Can you work these out from the model? Positions are in its coordinate system, mm. Face numbers are marked on the shaded views. A direction names the side the tool comes from. Give positions to 0.01 mm unless a question says otherwise; leave off trailing zeros. Order: outer loops, then holes, each group sorted by start corner. A loop starts at its lowest first (then second) coordinate and runs counter-clockwise, first axis right, second up. Notation, with made-up numbers: (-11, 75) - (36, 75) arc R22 ccw to (36, 99) - close; hole circle Ø7 at (2, 46.5). An arc over 180 degrees is marked (long way). Answer as CSV lines item,"result".
```python
from build123d import *

# Parameters (mm, degrees)
SKETCH1_R           = 1
BOSS_EXTRUDE1_DEPTH = 3
SKETCH2_W           = 15
SKETCH2_H           = 25
CUT_EXTRUDE1_DEPTH  = 1
SKETCH3_W           = 15
SKETCH3_H           = 25
CUT_EXTRUDE2_DEPTH  = 1


with BuildPart() as part:
    # Sketch1 → Boss-Extrude1 (new body)
    with BuildSketch(Plane(origin=(0, 0, 0), x_dir=(1, 0, 0), z_dir=(0, 1, 0))):
        with BuildLine():
            Line((-52.254901961, 26.274509804), (-12.254901961, 26.274509804))
            ThreePointArc((-12.254901961, 26.274509804), (-8.719368055, 24.81004371), (-7.254901961, 21.274509804))
            Line((-7.254901961, 21.274509804), (-7.254901961, -28.725490196))
            ThreePointArc((-7.254901961, -28.725490196), (-8.719368055, -32.261024102), (-12.254901961, -33.725490196))
            Line((-12.254901961, -33.725490196), (-52.254901961, -33.725490196))
            ThreePointArc((-52.254901961, -33.725490196), (-55.790435867, -32.261024102), (-57.254901961, -28.725490196))
            Line((-57.254901961, -28.725490196), (-57.254901961, 21.274509804))
            ThreePointArc((-57.254901961, 21.274509804), (-55.790435867, 24.81004371), (-52.254901961, 26.274509804))
        make_face()
        with Locations(Location((-32.254901961, -3.725490196, 0), (0, 0, 270))):
            Circle(SKETCH1_R, mode=Mode.SUBTRACT)
        with Locations(Location((-47.254901961, 3.774509804, 0), (0, 0, 270))):
            Circle(SKETCH1_R, mode=Mode.SUBTRACT)
        with Locations(Location((-47.254901961, -11.225490196, 0), (0, 0, 270))):
            Circle(SKETCH1_R, mode=Mode.SUBTRACT)
        with Locations(Location((-17.254901961, 3.774509804, 0), (0, 0, 270))):
            Circle(SKETCH1_R, mode=Mode.SUBTRACT)
        with Locations(Location((-17.254901961, -11.225490196, 0), (0, 0, 270))):
            Circle(SKETCH1_R, mode=Mode.SUBTRACT)
    extrude(amount=BOSS_EXTRUDE1_DEPTH)

    # Sketch2 → Cut-Extrude1 (cut)
    with BuildSketch(Plane(origin=(0, 3, 0), x_dir=(1, 0, 0), z_dir=(0, 1, 0))):
        with Locations((-49.754901961, -3.725490196)):
            Rectangle(SKETCH2_W, SKETCH2_H)
    extrude(amount=-CUT_EXTRUDE1_DEPTH, mode=Mode.SUBTRACT)

    # Sketch3 → Cut-Extrude2 (cut)
    with BuildSketch(Plane(origin=(0, 3, 0), x_dir=(1, 0, 0), z_dir=(0, 1, 0))):
        with Locations((-14.754901961, -3.725490196)):
            Rectangle(SKETCH3_W, SKETCH3_H)
    extrude(amount=-CUT_EXTRUDE2_DEPTH, mode=Mode.SUBTRACT)


solid = part.part
```
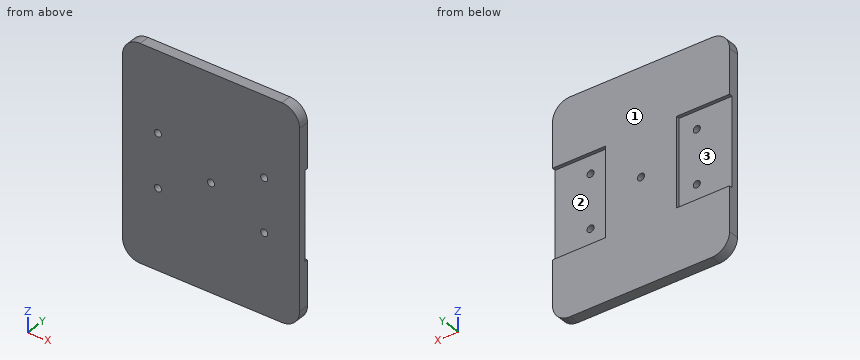
1) Which directions (+Z, -Z, +X, -X, +Y, -Y) give clear straight access to the entire face, cutting with the end or side of a thin tool? Please do the marked faces 1, 2 and 3.
Answer block:
face 1,"+Z, -Z, +X, -X, +Y"
face 2,"+X, +Y"
face 3,"-X, +Y"
2) I need wall thicknesses on line 1 along Z through (x, y) = (-17, 2.6); line 2 along X through (y, z) = (2.1, -8.5); line 3 along Z through (x, y) = (-46.5, 0.7). Which ranges of each line are inside material? Lowest first, please. Write a range as [from, to].
Answer block:
line 1,"[-26.27, -8.77], [16.23, 33.73]"
line 2,"[-42.25, -22.25]"
line 3,"[-26.27, -4.43], [-3.12, 10.57], [11.88, 33.73]"
3) I want a section at B-B on x = -49.5. Write out the boundary of the cut face in (y, z), plus the area to 3 significant figures.
Answer block:
outline,"(0, -26.27) - (3, -26.27) - (3, -8.77) - (2, -8.77) - (2, 16.23) - (3, 16.23) - (3, 33.73) - (0, 33.73) - close"
area,"155 mm2"
4) I want a section at C-C on y = 2.5. Write out the boundary of the cut face in (x, z), plus the area to 3 significant figures.
Answer block:
outline,"(-57.25, -21.27) arc R5 ccw to (-52.25, -26.27) - (-12.25, -26.27) arc R5 ccw to (-7.25, -21.27) - (-7.25, -8.77) - (-22.25, -8.77) - (-22.25, 16.23) - (-7.25, 16.23) - (-7.25, 28.73) arc R5 ccw to (-12.25, 33.73) - (-52.25, 33.73) arc R5 ccw to (-57.25, 28.73) - (-57.25, 16.23) - (-42.25, 16.23) - (-42.25, -8.77) - (-57.25, -8.77) - close; hole circle Ø2 at (-32.25, 3.73)"
area,"2,230 mm2"
5) I want a section at A-A on z = 9.5. Write out the boundary of the cut face in (x, y), plus the area to 3 significant figures.
Answer block:
outline,"(-57.25, 0) - (-7.25, 0) - (-7.25, 2) - (-22.25, 2) - (-22.25, 3) - (-42.25, 3) - (-42.25, 2) - (-57.25, 2) - close"
area,"120 mm2"
6) I'm going to push a flat-ended pin straight in: P1, Ø7.5, axis at x = -52.5, z = -1, coming from the +Y side. Where does the tip first touch, or does it pass through?
Answer block:
P1,"y = 2"
